from build123d import *

# Parameters (mm, degrees)
SKETCH1_R               = 1.5
BOSS_EXTRUDE1_DEPTH     = 7
FILLET1_R               = 2
FILLET2_R               = 4
SHELL1_T                = -1
CUT_EXTRUDE1_DEPTH      = 65.079559318
CUT_EXTRUDE1_DEPTH_BACK = 65.079559318
SKETCH3_W               = 7
SKETCH3_H               = 14
CUT_EXTRUDE2_DEPTH      = 2


with BuildPart() as part:
    # Sketch1 → Boss-Extrude1 (new, symmetric)
    with BuildSketch(Plane.XY):
        Polygon((4, 4.3), (-63, 4.3), (-63, -9.7), (5.2, -4.619641248), align=None)
        Circle(SKETCH1_R, mode=Mode.SUBTRACT)
        with Locations((-59, -3)):
            Circle(SKETCH1_R, mode=Mode.SUBTRACT)
    extrude(amount=BOSS_EXTRUDE1_DEPTH, both=True)

    # Fillet1
    fillet1_edges = [part.edges().sort_by_distance(p)[0] for p in [
        (-29.5, 4.3, 7),
        (-29.5, 4.3, -7),
    ]]
    fillet(fillet1_edges, radius=FILLET1_R)

    # Fillet2
    fillet2_edges = [part.edges().sort_by_distance(p)[0] for p in [
        (-63, -9.7, 0),
        (5.2, -4.619641248, 0),
    ]]
    fillet(fillet2_edges, radius=FILLET2_R)

    # Shell1
    shell1_openings = [part.faces().sort_by_distance(p)[0] for p in [
        (-60.5, -3, 0),
        (-1.5, 0, 0),
        (-61.721343434, -8.3225509, 0),
        (3.776615154, -3.465411477, 0),
        (-63, -0.601849653, 0),
        (4.323873752, 1.892635268, 0),
        (-28.867987445, -7.157435943, 0),
    ]]
    offset(amount=SHELL1_T, openings=shell1_openings, kind=Kind.INTERSECTION)

    # Sketch2 → Cut-Extrude1 (cut, two sides: drawn at the far end of the back side and taken through both)
    with BuildSketch(Plane.XY.offset(-CUT_EXTRUDE1_DEPTH_BACK)):
        Polygon((-43, -8.210158724), (-41, -5.303555184), (-31.027630399, -4.560692791), (-29.027630399, -7.169328076), align=None)
    extrude(amount=CUT_EXTRUDE1_DEPTH + CUT_EXTRUDE1_DEPTH_BACK, mode=Mode.SUBTRACT)

    # Sketch3 → Cut-Extrude2 (cut)
    with BuildSketch(Plane(origin=(0, 4.3, 0), x_dir=(1, 0, 0), z_dir=(0, 1, 0))):
        with Locations((1.134020196, 0)):
            Rectangle(SKETCH3_W, SKETCH3_H)
    extrude(amount=-CUT_EXTRUDE2_DEPTH, mode=Mode.SUBTRACT)


solid = part.part
Geometry: final body of the model. Coordinates: model frame, mm. A direction names the side the tool comes from. Round coordinates to 2 decimals unless told otherwise and drop trailing zeros. Loops run counter-clockwise (first coordinate to the right, second up) from the corner with the lowest first, then second, coordinate; pieces in that order, holes last. Notation, with made-up numbers: M -14.75,26 L 18.25,26 A29 ccw 18.25,61 Z; hole C 5,48.5 d7. An arc over 180 degrees is marked long. Put each result on its own line as item: value. Start each with the question number.
(1) Section query D-D (x = -47). Return loops of the section in (y, z), then the cut area to 3 significant figures.
(2) Section query C-C (z = 0.5). Return loops of the section in (x, y), then the cut area to 3 significant figures.
(3) Contact query for flat-ended pins moving along their axis: pin 1 Ø1 at (x, y) = (-11.5, -6) entering from -Z; pin 2 Ø0.5 at (x, z) = (0.5, 6.5) entering from +Y; pin 3 Ø2 at (y, z) = (-7.5, -5.5) entering from -X; pin 4 Ø2 at (y, z) = (3.5, -3.5) entering from +X. Output: stop coordinate, or through.
(4) Set-up query: faces 1 (the face through (-30.04, -5.85, -6.51)), 2 (the face through (-50.961, -8.803, 6.507)), 3 (the face through (-30, -2, 6)). Return all of +Z, -Z, +X, -X, +Y, -Y with unobstructed straight access to the full face (end or side cutting, diameter ignored); none if empty.
(5) Draft query along Z for faces 4 (the face through (-32, 4.3, 0)), 5 (the face through (-32, 3.3, 0)), 6 (the face through (-30, -2, 7)). Return one class per face: +Z half, -Z half, draft (parallel to the pull), parting line (faces both ways), or undercut.
(6) Section query B-B (y = -3). Return loops of the section in (x, z), then the cut area to 3 significant figures.
(7) Material intervals for line 1 along Z through (x, y) = (-54, -7); line 2 along Y through (x, z) = (0, 6.4); line 3 along X through (y, z) = (-3, -6.15), sorted ascending. Write a range as [from, to].
(8) Section query A-A (x = 0). Return loops of the section in (y, z), then the cut area to 3 significant figures.
Findings below:
1. outline: M -8.51,-7 L 2.3,-7 A2 ccw 4.3,-5 L 4.3,5 A2 ccw 2.3,7 L -8.51,7 L -8.51,6 L 2.3,6 A1 cw 3.3,5 L 3.3,-5 A1 cw 2.3,-6 L -8.51,-6 Z
1. area: 36.3 mm2
2. outline: M -63,3.3 L -2.37,3.3 L -2.37,4.3 L -63,4.3 Z
2. area: 60.6 mm2
3. pin 1: stops at z = -7
3. pin 2: stops at y = 2.3
3. pin 3: stops at x = -62.8
3. pin 4: stops at x = -2.37
4. face 1: +Z, -Z, -Y
4. face 2: +Z, -Z, +X, -Y
4. face 3: +X, -X, -Y
5. face 4: draft
5. face 5: undercut
5. face 6: +Z half
6. outline: M -63,-7 L -60.5,-7 L -60.5,-6 L -63,-6 Z; M -63,6 L -60.5,6 L -60.5,7 L -63,7 Z; M -57.5,-7 L 4.1,-7 L 4.1,-6 L -57.5,-6 Z; M -57.5,6 L 4.1,6 L 4.1,7 L -57.5,7 Z
6. area: 128 mm2
7. line 1: z = [-7, -6], [6, 7]
7. line 2: y = [-5.01, -1.5], [1.5, 2.3]
7. line 3: x = [-63, -60.5], [-57.5, 4.1]
8. outline: M -5.01,-7 L -1.5,-7 L -1.5,-6 L -5.01,-6 Z; M -5.01,6 L -1.5,6 L -1.5,7 L -5.01,7 Z; M 1.5,-7 L 2.3,-7 L 2.3,-6 L 1.5,-6 Z; M 1.5,6 L 2.3,6 L 2.3,7 L 1.5,7 Z
8. area: 8.61 mm2
